The drawing under review shows one solid part. Ordinate dimensions are in mm from its lowest x, y, z. A direction names the side the tool comes from. Give positions to 0.01 mm unless a question says otherwise; leave off trailing zeros. Order: outer loops, then holes, each group sorted by start corner. A loop starts at its lowest first (then second) coordinate and runs counter-clockwise, first axis right, second up. Notation, with made-up numbers: (-32.5, 80) -> (-25.5, 80) arc R32 ccw to (-25.5, 116) -> close; hole circle Ø4 at (-8.5, -35). An arc over 180 degrees is marked (long way). Use CSV: the item, a comma, the result in double quotes. Start each with the question number.
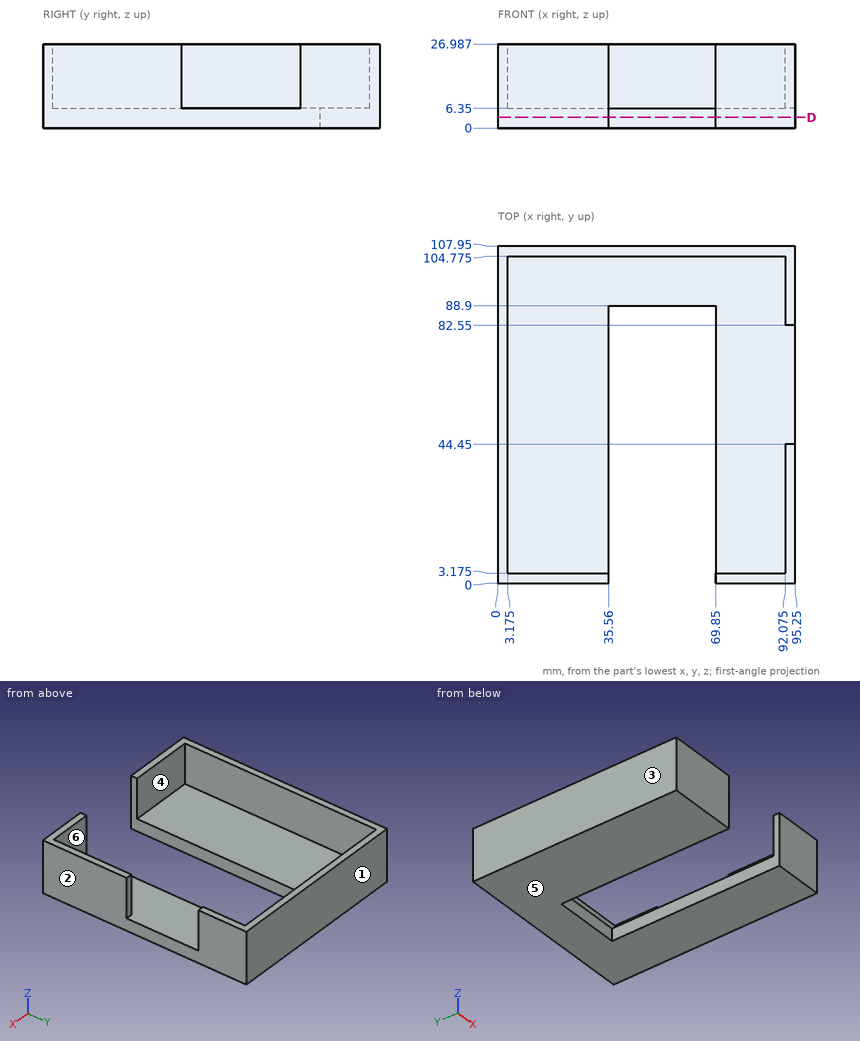
1. Consider section D-D (z = 3.5). State the section outline as (x, y) points.
2. For the marked faces 5 and 6, list the 3-axis set-ups (+Z, -Z, +X, -X, +Y, -Y) from which the entire face can be reached by the end or side of a thin tool; tool diameter is ignored.
3. Clearance check with flat-ended pins moving along their axes: P1, Ø5, axis at x = 51.5, z = 2.5, coming from the -Y side; P2, Ø6, axis at x = 40.5, z = 13, coming from the -Y side (1 decimal); P3, Ø6, axis at y = 68.5, z = 19.5, coming from the +X side (1 decimal). State where each tip first meets the part, or that it passes through.
4. To check wall thickness, follow L1, parallel to X at y = 31, z = 2; L2, parallel to Z at x = 82, y = 46.5; L3, parallel to X at y = 48.5, z = 9.75 (1 decimal). State the ranges of each line that lie inside material, in increasing order. Write a range as [from, to].
5. Draft analysis for pull direction X (two halves, no side actions). For the marked faces 1, 2, 3 and 4, state which applies: +X half, -X half, draft (parallel to the pull), parting line (faces both ways), or undercut.
Answer list:
1,outline,"(0, 0) -> (35.56, 0) -> (35.56, 88.9) -> (69.85, 88.9) -> (69.85, 0) -> (95.25, 0) -> (95.25, 107.95) -> (0, 107.95) -> close"
2,face 5,"-Z, +X, -X, +Y, -Y"
2,face 6,"+Z"
3,P1,"y = 88.9"
3,P2,"y = 104.8"
3,P3,"x = 3.2"
4,L1,"[0, 35.56], [69.85, 95.25]"
4,L2,"[0, 6.35]"
4,L3,"[0, 3.2]"
5,face 1,"draft"
5,face 2,"+X half"
5,face 3,"-X half"
5,face 4,"undercut"
